```python
from build123d import *

# Parameters (mm, degrees)
SKETCH1_W           = 18
SKETCH1_H           = 60
BOSS_EXTRUDE1_DEPTH = 16
SKETCH2_R           = 3.1
CUT_EXTRUDE1_DEPTH  = 36.17101079
SKETCH3_R           = 1.6
CUT_EXTRUDE2_DEPTH  = 39.470768123
SKETCH4_W           = 4
SKETCH4_H           = 14
BOSS_EXTRUDE2_DEPTH = 10
SKETCH5_R           = 1.6
CUT_EXTRUDE3_DEPTH  = 42.194659848
CHAMFER1_SIZE       = 3
BOSS_EXTRUDE3_DEPTH = 3
BOSS_EXTRUDE4_DEPTH = 3


with BuildPart() as part:
    # Sketch1 → Boss-Extrude1 (new body)
    with BuildSketch(Plane(origin=(0, 0, 0), x_dir=(1, 0, 0), z_dir=(0, 1, 0))):
        Rectangle(SKETCH1_W, SKETCH1_H)
    extrude(amount=BOSS_EXTRUDE1_DEPTH)

    # Sketch2 → Cut-Extrude1 (cut, through all)
    with BuildSketch(Plane(origin=(0, 16, 0), x_dir=(1, 0, 0), z_dir=(0, 1, 0))):
        with Locations(Location((0, 23, 0), (0, 0, 270))):
            Circle(SKETCH2_R)
        with Locations(Location((0, -23, 0), (0, 0, 270))):
            Circle(SKETCH2_R)
    extrude(amount=-CUT_EXTRUDE1_DEPTH, mode=Mode.SUBTRACT)

    # Sketch3 → Cut-Extrude2 (cut, through all)
    with BuildSketch(Plane.ZY.offset(9)):
        with Locations((-12, 8)):
            Circle(SKETCH3_R)
        with Locations((12, 8)):
            Circle(SKETCH3_R)
    extrude(amount=-CUT_EXTRUDE2_DEPTH, mode=Mode.SUBTRACT)

    # Sketch4 → Boss-Extrude2 (add)
    with BuildSketch(Plane(origin=(0, 16, 0), x_dir=(1, 0, 0), z_dir=(0, 1, 0))):
        Rectangle(SKETCH4_W, SKETCH4_H)
    extrude(amount=BOSS_EXTRUDE2_DEPTH)

    # Sketch5 → Cut-Extrude3 (cut, through all)
    with BuildSketch(Plane.ZY.offset(2)):
        with Locations((0, 21)):
            Circle(SKETCH5_R)
    extrude(amount=-CUT_EXTRUDE3_DEPTH, mode=Mode.SUBTRACT)

    # Chamfer1
    chamfer1_edges = [part.edges().sort_by_distance(p)[0] for p in [
        (0, 26, -7),
        (0, 26, 7),
    ]]
    chamfer(chamfer1_edges, length=CHAMFER1_SIZE)

    # Sketch6 → Boss-Extrude3 (add)
    with BuildSketch(Plane.XY.offset(7)):
        Polygon((-2, 18.5), (-4.5, 16), (-2, 16), align=None)
        Polygon((2, 18.5), (4.5, 16), (2, 16), align=None)
    extrude(amount=-BOSS_EXTRUDE3_DEPTH)

    # Sketch7 → Boss-Extrude4 (add)
    with BuildSketch(Plane(origin=(0, 0, -7), x_dir=(-1, 0, 0), z_dir=(0, 0, -1))):
        Polygon((2, 18.5), (2, 16), (4.5, 16), align=None)
        Polygon((-2, 16), (-2, 18.5), (-4.5, 16), align=None)
    extrude(amount=-BOSS_EXTRUDE4_DEPTH)


solid = part.part
```
Verification items for the finished model (mm, model axes). A direction names the side the tool comes from. Give positions to 0.01 mm unless a question says otherwise; leave off trailing zeros. Loops run counter-clockwise (first coordinate to the right, second up) from the corner with the lowest first, then second, coordinate; pieces in that order, holes last.
1. Section check B-B, the plane z = 0. Enter the section's corners in (x, y), then the cut area to 3 significant figures.
2. Thickness scan on line 1 (X direction, y = 7.25, z = 23); line 2 (Z direction, x = -2, y = 9.75); line 3 (Y direction, x = -4, z = 12). Record the ranges inside material, lowest first.
3. Section check D-D, the plane y = 3. Enter the section's corners in (x, z).
4. Set-up check for faces 1 (the flat face through (0, 19, 7)), 2 (the flat face through (2, 21, 2)), 3 (the flat face through (-3, 17, 4)), 4 (the flat face through (-9, 8, 0)): record each of +Z, -Z, +X, -X, +Y, -Y from which the full face is reachable in a straight line by a thin tool's end or side.
5. Mould release check, pull along Z, two halves, no side actions. Record for faces 5 (the flat face through (0, 8, 30)), 6 (the cylindrical face through (-0.028, 22.586, -0.208)), 7 (the flat face through (3, 17, -4)), 8 (the flat face through (-3.2, 17.3, 5.5)): released by +Z, released by -Z, zero draft, split by the parting line, or undercut.
6. Section check C-C, the plane y = 21. Enter the section's corners in (x, z).
7. Go/stop test with flat-tipped pins: pin 1 Ø3 at (y, z) = (8, 12) entering from -X; pin 2 Ø5 at (y, z) = (23, 1) entering from +X; pin 3 Ø0.8 at (x, y) = (-3, 17.5) entering from +Z; pin 4 Ø5 at (y, z) = (21, 0) entering from -X. Record where each tip stops, or that it passes through.
8. Section check A-A, the plane x = 0. Enter the section's corners in (y, z), then the cut area to 3 significant figures.
Geometry says:
1. outline: (-9, 0) - (9, 0) - (9, 16) - (2, 16) - (2, 19.4) - (-2, 19.4) - (-2, 16) - (-9, 16) - close; (-2, 22.6) - (2, 22.6) - (2, 26) - (-2, 26) - close
1. area: 315 mm2
2. line 1: x = -9 to -3.1, 3.1 to 9
2. line 2: z = -30 to -25.37, -20.63 to 20.63, 25.37 to 30
2. line 3: y = 0 to 6.4, 9.6 to 16
3. outline: (-9, -30) - (9, -30) - (9, 30) - (-9, 30) - close; hole circle Ø6.2 at (0, -23); hole circle Ø6.2 at (0, 23)
4. face 1: +Z, +X, -X, +Y
4. face 2: +X, +Y
4. face 3: -X, +Y
4. face 4: +Z, -Z, -X, +Y, -Y
5. face 5: released by +Z
5. face 6: undercut
5. face 7: undercut
5. face 8: zero draft
6. outline: (-2, -7) - (2, -7) - (2, -1.6) - (-2, -1.6) - close; (-2, 1.6) - (2, 1.6) - (2, 7) - (-2, 7) - close
7. pin 1: passes through
7. pin 2: stops at x = 2
7. pin 3: stops at z = 7
7. pin 4: stops at x = -2
8. outline: (0, -30) - (16, -30) - (16, -26.1) - (0, -26.1) - close; (0, -19.9) - (16, -19.9) - (16, -7) - (23, -7) - (26, -4) - (26, 4) - (23, 7) - (16, 7) - (16, 19.9) - (0, 19.9) - close; (0, 26.1) - (16, 26.1) - (16, 30) - (0, 30) - close; hole circle Ø3.2 at (8, -12); hole circle Ø3.2 at (8, 12); hole circle Ø3.2 at (21, 0)
8. area: 868 mm2
